Study the drawing (mm; zero at the part's minimum x, y, z) and answer. Coordinates: 2 decimals unless noted, no trailing zeros. Loops run counter-clockwise (first coordinate to the right, second up) from the corner with the lowest first, then second, coordinate; pieces in that order, holes last. Notation, with made-up numbers: (57, 88) -> (82, 88) arc R13 ccw to (82, 102) -> close; hole circle Ø4 at (36.5, 89.25). An arc over 180 degrees is marked (long way). Answer as a JSON object with one key per item and string values. Group by question number.
Q1. Each of these flat-tipped pins is pushed along its axis until it touches: P1, Ø4.5, axis at x = 7.5, y = 25, coming from the -Z side; P2, Ø0.6, axis at y = 56, z = 1, coming from the +X side; P3, Ø1, axis at y = 57.5, z = 0.5, coming from the -X side; P4, Ø3.5, axis at x = 25, y = 42.5, coming from the +Z side. Where does it stop, or does it pass through?
Q2. The part is cut by section D-D on x = 7.5. Write down the section's boundary in (y, z), and give its area (3 significant figures).
Q3. The part is cut by section B-B on z = 0.8. Write down the section's boundary in (x, y).
Q4. Straight lines are drawn through the part: line 1 along Y through (x, z) = (25, 1); line 2 along X through (y, z) = (57, 0.9); line 3 along Y through (x, z) = (25.5, 0.4) (1 decimal). For each, find the intervals that lie inside material, in ascending order. Write a range as [from, to].
Q5. The part is cut by section A-A on x = 25. Write down the section's boundary in (y, z), and give its area (3 significant figures).
Q6. The part is cut by section C-C on y = 17. Write down the section's boundary in (x, z).
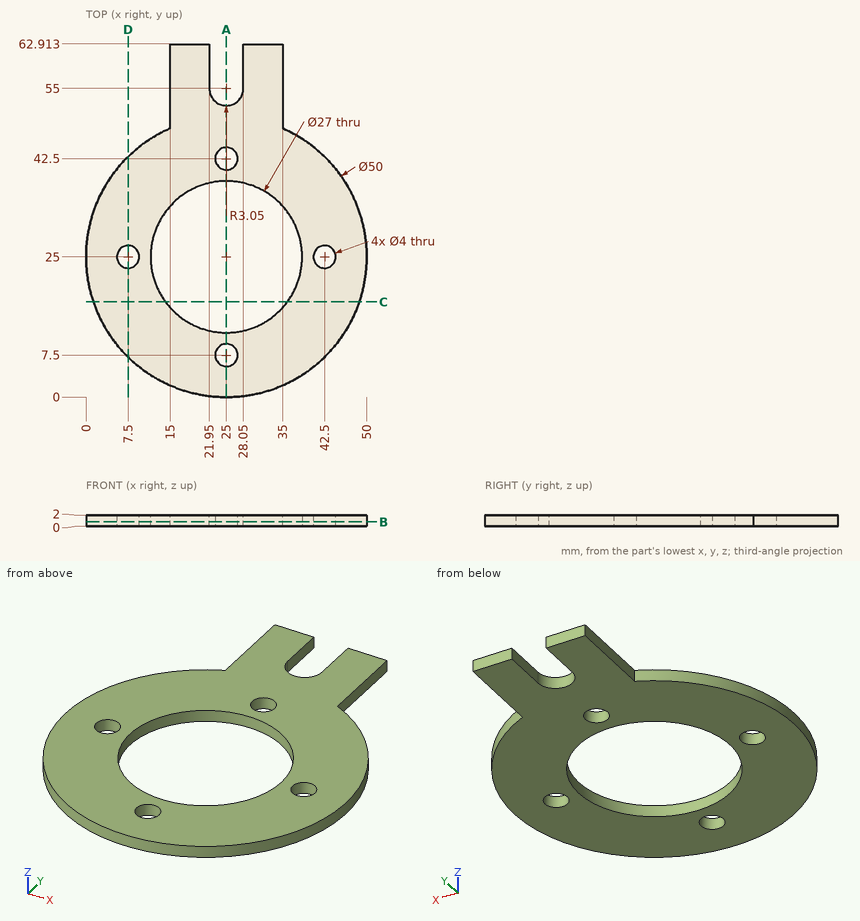
Final values:
{
 "1": {"P1": "stops at z = 0", "P2": "stops at x = 35", "P3": "stops at x = 15", "P4": "passes through"},
 "2": {"outline": "(7.15, 0) -> (23, 0) -> (23, 2) -> (7.15, 2) -> close; (27, 0) -> (42.85, 0) -> (42.85, 2) -> (27, 2) -> close", "area": "63.4 mm2"},
 "3": {"outline": "(15, 47.91) arc R25 ccw (long way) to (35, 47.91) -> (35, 62.91) -> (28.05, 62.91) -> (28.05, 55) arc R3.05 cw to (21.95, 55) -> (21.95, 62.91) -> (15, 62.91) -> close; hole circle Ø4 at (7.5, 25); hole circle Ø27 at (25, 25); hole circle Ø4 at (25, 7.5); hole circle Ø4 at (25, 42.5); hole circle Ø4 at (42.5, 25)"},
 "4": {"line 1": "y = [0, 5.5], [9.5, 11.5], [38.5, 40.5], [44.5, 51.95]", "line 2": "x = [15, 21.95], [28.05, 35]", "line 3": "y = [0, 5.6], [9.4, 11.5], [38.5, 40.6], [44.4, 52]"},
 "5": {"outline": "(0, 0) -> (5.5, 0) -> (5.5, 2) -> (0, 2) -> close; (9.5, 0) -> (11.5, 0) -> (11.5, 2) -> (9.5, 2) -> close; (38.5, 0) -> (40.5, 0) -> (40.5, 2) -> (38.5, 2) -> close; (44.5, 0) -> (51.95, 0) -> (51.95, 2) -> (44.5, 2) -> close", "area": "33.9 mm2"},
 "6": {"outline": "(1.31, 0) -> (14.13, 0) -> (14.13, 2) -> (1.31, 2) -> close; (35.87, 0) -> (48.69, 0) -> (48.69, 2) -> (35.87, 2) -> close"}
}
